Source: three-view drawing plus pictorial views. Frame: mm from the lowest corner of the part. A direction names the side the tool comes from. Round coordinates to 2 decimals unless told otherwise and drop trailing zeros. Write each loop counter-clockwise with the first axis right and the second up, starting at its lowest first coordinate (ties: lowest second). Pieces come first, ordered by that corner, then holes.
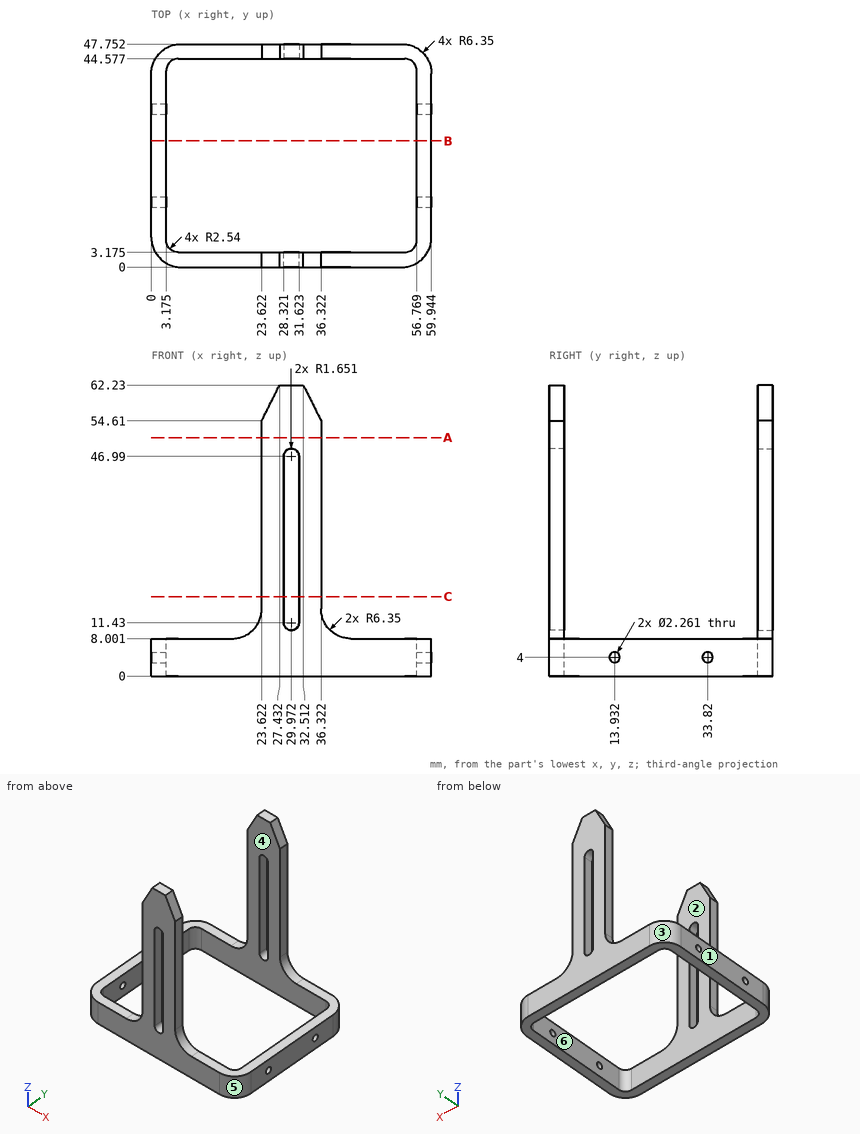
1) Section B-B on y = 27. Output: boundary loops of the cut face in (x, z) (1 decimal).
2) Section A-A on z = 51. Output: boundary loops of the cut face in (x, y) (1 decimal).
3) Line query: probe 1 along X at (y, z) = (45, 43.5); probe 2 along Y at (x, z) = (33.5, 6.5) (1 decimal); probe 3 along Z at (x, y) = (57, 44.5). Output: solid intervals per line, ascending.
4) Reachability of the marked faces 5 and 6 from +Z, -Z, +X, -X, +Y, -Y: full face, straight path, thin tool, end or side. Return the list, or none.
5) Draft query along Y for the marked faces 1, 2, 3 and 4. Return one class per face: pulls with the +Y half, pulls with the -Y half, needs draft (parallel to the pull), parting line crosses it, or undercut.
6) First-contact query: P1, Ø1, axis at y = 45.5, z = 27.5, coming from the +X side; P2, Ø3.5, axis at y = 46.5, z = 24.5, coming from the -X side. Flat tips, straight axial feed; report the tip coordinate or a pass-through.
7) Section C-C on z = 17. Output: boundary loops of the cut face in (x, y) (1 decimal).
Filled in:
1. outline: (0, 0) - (3.2, 0) - (3.2, 8) - (0, 8) - close; (56.8, 0) - (59.9, 0) - (59.9, 8) - (56.8, 8) - close
2. outline: (23.6, 0) - (36.3, 0) - (36.3, 3.2) - (23.6, 3.2) - close; (23.6, 44.6) - (36.3, 44.6) - (36.3, 47.8) - (23.6, 47.8) - close
3. probe 1: x = 23.62 to 28.32, 31.62 to 36.32
3. probe 2: y = 0 to 3.2, 44.6 to 47.8
3. probe 3: z = 0 to 8
4. face 5: +Z, -Z, +X, -Y
4. face 6: +Z, -Z
5. face 1: needs draft
5. face 2: undercut
5. face 3: pulls with the +Y half
5. face 4: undercut
6. P1: stops at x = 36.32
6. P2: stops at x = 23.62
7. outline: (23.6, 0) - (28.3, 0) - (28.3, 3.2) - (23.6, 3.2) - close; (23.6, 44.6) - (28.3, 44.6) - (28.3, 47.8) - (23.6, 47.8) - close; (31.6, 0) - (36.3, 0) - (36.3, 3.2) - (31.6, 3.2) - close; (31.6, 44.6) - (36.3, 44.6) - (36.3, 47.8) - (31.6, 47.8) - close
